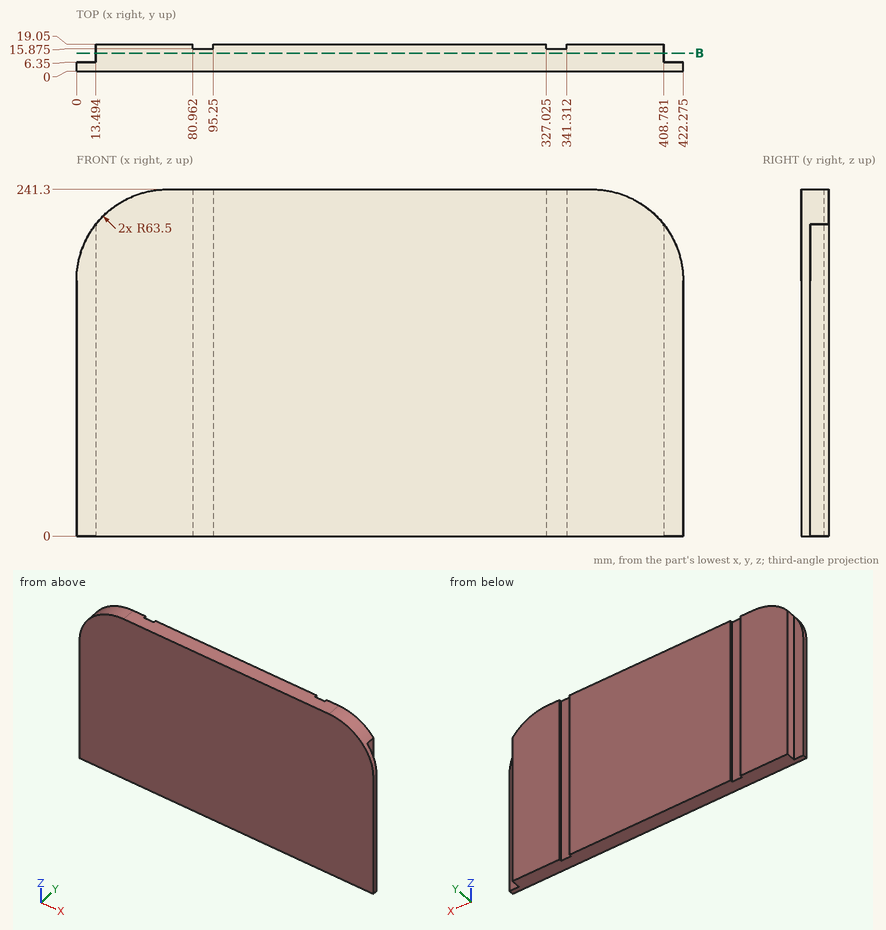
Geometry check sheet. Reference: drawing and pictorial views, mm from the part's lowest x, y, z. Coordinates: 2 decimals unless noted, no trailing zeros. Order: outer loops, then holes, each group sorted by start corner. A loop starts at its lowest first (then second) coordinate and runs counter-clockwise, first axis right, second up.
1. Go/stop test with flat-tipped pins: pin 1 Ø8 at (y, z) = (16.5, 164) entering from -X; pin 2 Ø1 at (y, z) = (14, 198.5) entering from +X; pin 3 Ø11 at (x, z) = (7.5, 88.5) entering from +Y; pin 4 Ø10 at (y, z) = (10, 112) entering from +X (1 decimal). Record where each tip stops, or that it passes through.
Results found:
pin 1: stops at x = 13.49
pin 2: stops at x = 408.78
pin 3: stops at y = 6.35
pin 4: stops at x = 422.3
2. Scan lines: line 1 (X direction, y = 9.25, z = 176.5); line 2 (Z direction, x = 28, y = 12.25); line 3 (Z direction, x = 386, y = 2). Record each from-to range of solid material in increasing order.
Results found:
line 1: x = 13.49 to 408.78
line 2: z = 0 to 230.45
line 3: z = 0 to 235.17
3. Sectioned sample at B-B, the plane y = 12.75. Record the cut outline in (x, z) (1 decimal).
Results found:
outline: (13.5, 0) - (408.8, 0) - (408.8, 216.9) arc R63.5 ccw to (358.8, 241.3) - (63.5, 241.3) arc R63.5 ccw to (13.5, 216.9) - close
